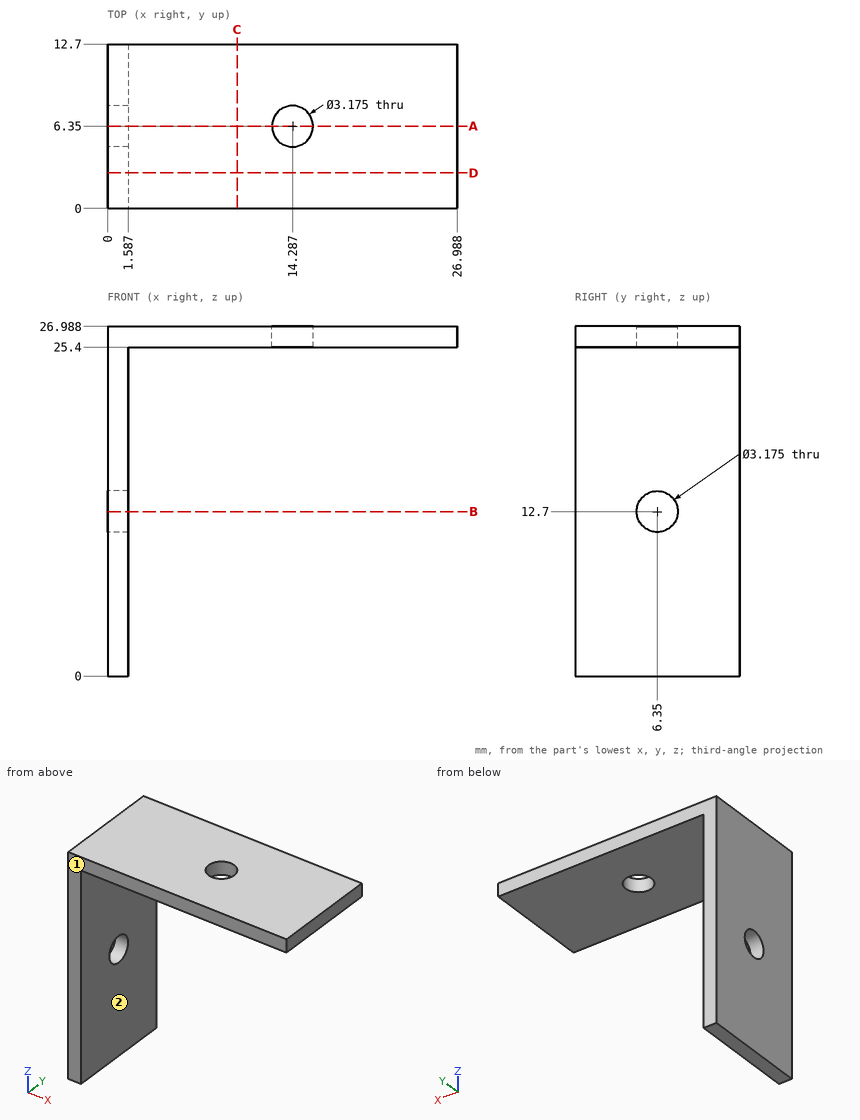
Geometry: see drawing. Coordinates: mm, zero at the bounding-box minimum. A direction names the side the tool comes from. Coordinates: 2 decimals unless noted, no trailing zeros. Write each loop counter-clockwise with the first axis right and the second up, starting at its lowest first coordinate (ties: lowest second). Pieces come first, ordered by that corner, then holes.
1) Section C-C on x = 10. Output: boundary loops of the cut face in (y, z).
2) Section B-B on z = 12.7. Output: boundary loops of the cut face in (x, y).
3) Section A-A on y = 6.35. Output: boundary loops of the cut face in (x, z) (1 decimal).
4) Set-up query: the marked faces 1 and 2. Return all of +Z, -Z, +X, -X, +Y, -Y with unobstructed straight access to the full face (end or side cutting, diameter ignored); none if empty.
5) Section D-D on y = 2.75. Output: boundary loops of the cut face in (x, z).
6) Material intervals for line 1 along Z through (x, y) = (0.65, 6.35); line 2 along Y through (x, z) = (0.65, 12.7); line 3 along X through (y, z) = (6.35, 26) (1 decimal), sorted ascending.
7) Pin query (flat end, axial travel): pin 1 Ø4 at (x, y) = (20, 10.5) entering from -Z. Return the tip coordinate at first contact, or that it passes through.
Check result:
1. outline: (0, 25.4) - (12.7, 25.4) - (12.7, 26.99) - (0, 26.99) - close
2. outline: (0, 0) - (1.59, 0) - (1.59, 4.76) - (0, 4.76) - close; (0, 7.94) - (1.59, 7.94) - (1.59, 12.7) - (0, 12.7) - close
3. outline: (0, 0) - (1.6, 0) - (1.6, 11.1) - (0, 11.1) - close; (0, 14.3) - (1.6, 14.3) - (1.6, 25.4) - (12.7, 25.4) - (12.7, 27) - (0, 27) - close; (15.9, 25.4) - (27, 25.4) - (27, 27) - (15.9, 27) - close
4. face 1: +Z, -Z, +X, -X, -Y
4. face 2: -Z, +X, +Y, -Y
5. outline: (0, 0) - (1.59, 0) - (1.59, 25.4) - (26.99, 25.4) - (26.99, 26.99) - (0, 26.99) - close
6. line 1: z = 0 to 11.11, 14.29 to 26.99
6. line 2: y = 0 to 4.76, 7.94 to 12.7
6. line 3: x = 0 to 12.7, 15.9 to 27
7. pin 1: stops at z = 25.4
